```python
from build123d import *

# Parameters (mm, degrees)
EXTRUDE_1_DEPTH     = 38
SKETCH_2_W          = 60
SKETCH_2_H          = 34
CUT_EXTRUDE_1_DEPTH = 13
SKETCH_3_R          = 5
SKETCH_3_W          = 2.616489735
SKETCH_3_H          = 10.586779654
SKETCH_3_W_2        = 2.616489734
CUT_EXTRUDE_4_DEPTH = 31
SKETCH_4_W          = 2
SKETCH_4_H          = 75.8952895
EXTRUDE_3_DEPTH     = 4
SKETCH_5_W          = 5.94764475
SKETCH_5_H          = 8
CUT_EXTRUDE_5_DEPTH = 4
SKETCH_6_W          = 64
SKETCH_6_H          = 8
EXTRUDE_4_DEPTH     = 3


with BuildPart() as part:
    # 草图1 → 凸台-拉伸1 (new body)
    with BuildSketch(Plane(origin=(0, 0, 0), x_dir=(1, 0, 0), z_dir=(0, 1, 0))):
        Polygon((-2, 75.8952895), (0, 75.8952895), (0, 69.94764475), (6.11103449, 69.94764475), (6.11103449, 5.94764475), (0, 5.94764475), (0, 0), (-2, 0), (-2, 5.94764475), (-8.11103449, 5.94764475), (-8.11103449, 69.94764475), (-2, 69.94764475), align=None)
    extrude(amount=EXTRUDE_1_DEPTH)

    # 草图2 → 切除-拉伸1 (cut)
    with BuildSketch(Plane(origin=(6.11103449, 0, 0), x_dir=(0, 0, -1), z_dir=(1, 0, 0))):
        with Locations((37.94764475, 19)):
            Rectangle(SKETCH_2_W, SKETCH_2_H)
    extrude(amount=-CUT_EXTRUDE_1_DEPTH, mode=Mode.SUBTRACT)

    # 草图3 → 切除-拉伸4 (cut)
    with BuildSketch(Plane.ZY.offset(8.11103449)):
        with Locations((-53.94764475, 28.5)):
            Circle(SKETCH_3_R)
        with Locations((-63.098105483, 10.137074157)):
            Rectangle(SKETCH_3_W, SKETCH_3_H)
        with Locations((-47.413673753, 10.137074157)):
            Rectangle(SKETCH_3_W, SKETCH_3_H)
        with BuildLine():
            ThreePointArc((-46.105428885, 28.079391153), (-29.781734116, 28.710374202), (-46.116264816, 28.5))
            Line((-46.116264816, 28.5), (-46.105428885, 28.5))
            Line((-46.105428885, 28.5), (-46.105428885, 28.079391153))
        make_face()
        with Locations((-28.470779817, 10.143507991)):
            Rectangle(SKETCH_3_W, SKETCH_3_H)
        with Locations((-53.94764475, 9.5)):
            Rectangle(SKETCH_3_W_2, SKETCH_3_H)
        with Locations((-21.94764475, 28.5)):
            Circle(SKETCH_3_R)
        with Locations((-12.808019949, 10.143507991)):
            Rectangle(SKETCH_3_W_2, SKETCH_3_H)
        with Locations((-21.94764475, 9.5)):
            Rectangle(SKETCH_3_W_2, SKETCH_3_H)
    extrude(amount=-CUT_EXTRUDE_4_DEPTH, mode=Mode.SUBTRACT)

    # 草图4 → 凸台-拉伸3 (add)
    with BuildSketch(Plane.XZ):
        with Locations((-1, -37.94764475)):
            Rectangle(SKETCH_4_W, SKETCH_4_H)
    extrude(amount=EXTRUDE_3_DEPTH)

    # 草图5 → 切除-拉伸5 (cut)
    with BuildSketch(Plane.ZY.offset(2)):
        with Locations((-72.921467125, 34)):
            Rectangle(SKETCH_5_W, SKETCH_5_H)
        with Locations((-2.973822375, 34)):
            Rectangle(SKETCH_5_W, SKETCH_5_H)
    extrude(amount=-CUT_EXTRUDE_5_DEPTH, mode=Mode.SUBTRACT)

    # 草图6 → 凸台-拉伸4 (add)
    with BuildSketch(Plane(origin=(6.11103449, 0, 0), x_dir=(0, 0, -1), z_dir=(1, 0, 0))):
        with Locations((37.94764475, 34)):
            Rectangle(SKETCH_6_W, SKETCH_6_H)
    extrude(amount=EXTRUDE_4_DEPTH)


solid = part.part
```
CAD build for the part. Positions are in the model's coordinates, mm. A direction names the side the tool comes from. Round coordinates to 2 decimals unless told otherwise and drop trailing zeros. Order: outer loops, then holes, each group sorted by start corner. A loop starts at its lowest first (then second) coordinate and runs counter-clockwise, first axis right, second up.
Item 1: Saw through at D-D on y = 6.5. State how many separate pieces and enclosed holes the cut face has, then the cut area to 3 significant figures.
Item 2: Pin check, flat tips, straight feed: pin 1 (0.6 mm diameter, centred on x = -7.5, y = 9.5, fed in from -Z); pin 2 (1.3 mm diameter, centred on x = -7.5, z = -22.5, fed in from -Y); pin 3 (0.6 mm diameter, centred on x = -7.5, y = 8.5, fed in from +Z). Stop position of each tip, or through.
Item 3: Tool access for faces 5 (the face through (-5, 0, -38)), 6 (the face through (0, 19, -7.948)), 7 (the face through (0, 2, -38)), 8 (the face through (8, 30, -37)): list every direction of +Z, -Z, +X, -X, +Y, -Y with a clear straight run to the whole face (end or side of a thin tool).
Item 4: Probe line 1 along Y through (x, z) = (5, -20.5); line 2 along Z through (x, y) = (1.5, 35); line 3 along Z through (x, y) = (-1, 28.5). List the from-to ranges inside material, lowest first.
Item 5: Saw through at A-A on y = 18.5. Write the cut outline in (x, z).
Item 6: Saw through at B-B on y = 32. Write the cut outline in (x, z), then the cut area to 3 significant figures.
Item 7: Saw through at C-C on z = -18.5. Write the cut outline in (x, y), then the cut area to 3 significant figures.
Item 8: Mould opens along X. For faces 1 (the face through (6.111, 1.6, -40.5)), 2 (the face through (3, 0, -38)), 3 (the face through (6.111, 33, -38)), 4 (the face through (0, 36, -54)) say: pulls with the +X half, pulls with the -X half, needs draft (parallel to the pull), parting line crosses it, or undercut.
Reported:
1. separate pieces: 7
1. enclosed holes: 0
1. area: 135 mm2
2. pin 1: stops at z = -69.95
2. pin 2: stops at y = 0
2. pin 3: stops at z = -5.95
3. face 5: +Z, -Z, -X, -Y
3. face 6: none
3. face 7: +X
3. face 8: +Z, -Z, +X, -Y
4. line 1: y = 0 to 2, 36 to 38
4. line 2: z = -69.95 to -67.95, -7.95 to -5.95
4. line 3: z = -75.9 to -67.95, -7.95 to 0
5. outline: (-8.11, -69.95) - (-2, -69.95) - (-2, -75.9) - (0, -75.9) - (0, -69.95) - (6.11, -69.95) - (6.11, -67.95) - (-6.89, -67.95) - (-6.89, -7.95) - (6.11, -7.95) - (6.11, -5.95) - (0, -5.95) - (0, 0) - (-2, 0) - (-2, -5.95) - (-8.11, -5.95) - close
6. outline: (-8.11, -69.95) - (9.11, -69.95) - (9.11, -5.95) - (-8.11, -5.95) - (-8.11, -18.38) - (-6.89, -18.38) - (-6.89, -7.95) - (6.11, -7.95) - (6.11, -67.95) - (-6.89, -67.95) - (-6.89, -57.52) - (-8.11, -57.52) - close; (-8.11, -50.38) - (-6.89, -50.38) - (-6.89, -45.33) - (-8.11, -45.33) - close; (-8.11, -30.57) - (-6.89, -30.57) - (-6.89, -25.52) - (-8.11, -25.52) - close
6. area: 287 mm2
7. outline: (-8.11, 0) - (-2, 0) - (-2, -4) - (0, -4) - (0, 0) - (6.11, 0) - (6.11, 2) - (-6.89, 2) - (-6.89, 24.88) - (-8.11, 24.88) - close; (-8.11, 32.12) - (-6.89, 32.12) - (-6.89, 36) - (6.11, 36) - (6.11, 30) - (9.11, 30) - (9.11, 38) - (-8.11, 38) - close
7. area: 122 mm2
8. face 1: pulls with the +X half
8. face 2: needs draft
8. face 3: undercut
8. face 4: undercut
